Build history of the part. All positions in model axes, mm. A direction names the side the tool comes from. Give positions to 0.01 mm unless a question says otherwise; leave off trailing zeros. Order: outer loops, then holes, each group sorted by start corner. A loop starts at its lowest first (then second) coordinate and runs counter-clockwise, first axis right, second up. Notation, with made-up numbers: (49.5, 13) -> (68.5, 13) arc R11 cw to (68.5, 18) -> close; hole circle Ø11 at (-27, 19). An arc over 180 degrees is marked (long way). Write item = value, one per line. Start each with the question number.
from build123d import *

# Parameters (mm, degrees)
SKETCH013_R                          = 1.25
EXTRUDE009_DEPTH                     = 12
SKETCH012_R                          = 1.25
EXTRUDE008_DEPTH                     = 15
SKETCH011_W                          = 40
SKETCH011_H                          = 25
EXTRUDE007_DEPTH                     = 5
SKETCH010_W                          = 40
SKETCH010_H                          = 25
EXTRUDE006_DEPTH                     = 2
EXTRUDE004_DEPTH                     = 18
EXTRUDE004_ONTO_SKETCH007_ROLL_ANGLE = 90
SKETCH006_AS_DRAWN_R                 = 12.5
EXTRUDE003_DEPTH                     = 65
EXTRUDE003_ONTO_SKETCH006_ROLL_ANGLE = 90
EXTRUDE002_DEPTH                     = 60
EXTRUDE002_ONTO_SKETCH005_ROLL_ANGLE = 90
SKETCH004_R                          = 1.65
EXTRUDE_DEPTH                        = 40
SKETCH_AS_DRAWN_W                    = 30
SKETCH_AS_DRAWN_H                    = 70
EXTRUDE001_DEPTH                     = 60
EXTRUDE001_ONTO_SKETCH_ROLL_ANGLE    = 90


with BuildPart() as extrude009:
    # Sketch013 → Extrude009 (new body)
    with BuildSketch(Plane.XY.offset(15)):
        with Locations((11.5, 56.5)):
            Circle(SKETCH013_R)
        with Locations((-11.5, 56.5)):
            Circle(SKETCH013_R)
    extrude(amount=EXTRUDE009_DEPTH)


with BuildPart() as extrude008:
    # Sketch012 → Extrude008 (new body)
    with BuildSketch(Plane.XY.offset(70)):
        with Locations((0, 47)):
            Circle(SKETCH012_R)
        with Locations((11.5, 56.5)):
            Circle(SKETCH012_R)
        with Locations((-11.5, 56.5)):
            Circle(SKETCH012_R)
    extrude(amount=-EXTRUDE008_DEPTH)


with BuildPart() as extrude007:
    # Sketch011 → Extrude007 (new body)
    with BuildSketch(Plane(origin=(0, 35, 16), x_dir=(1, 0, 0), z_dir=(0, 0, 1))):
        with Locations((0, 20)):
            Rectangle(SKETCH011_W, SKETCH011_H)
    extrude(amount=-EXTRUDE007_DEPTH)


with BuildPart() as extrude006:
    # Sketch010 → Extrude006 (new body)
    with BuildSketch(Plane(origin=(0, 35, 70), x_dir=(1, 0, 0), z_dir=(0, 0, 1))):
        with Locations((0, 20)):
            Rectangle(SKETCH010_W, SKETCH010_H)
    extrude(amount=-EXTRUDE006_DEPTH)


with BuildPart() as extrude004:
    # Sketch007 as drawn → Extrude004 (new)
    with BuildSketch(Plane.XY):
        Polygon((17, 44), (7, 36), (7, 25), (17, 25), align=None)
        Polygon((-17, 44), (-7, 36), (-7, 25), (-17, 25), align=None)
    extrude(amount=-EXTRUDE004_DEPTH)


with BuildPart() as extrude004_1:
    # Extrude004 onto Sketch007 roll: moved
    add(extrude004.part.rotate(Axis((0, 0, 0), (1, 0, 0)), EXTRUDE004_ONTO_SKETCH007_ROLL_ANGLE))


with BuildPart() as extrude004_2:
    # Extrude004 onto Sketch007 placement: moved
    add(extrude004_1.part)


with BuildPart() as extrude003:
    # Sketch006 as drawn → Extrude003 (new)
    with BuildSketch(Plane.XY):
        with Locations((0, 50)):
            Circle(SKETCH006_AS_DRAWN_R)
    extrude(amount=-EXTRUDE003_DEPTH)


with BuildPart() as extrude003_1:
    # Extrude003 onto Sketch006 roll: moved
    add(extrude003.part.rotate(Axis((0, 0, 0), (1, 0, 0)), EXTRUDE003_ONTO_SKETCH006_ROLL_ANGLE))


with BuildPart() as extrude003_2:
    # Extrude003 onto Sketch006 placement: moved
    add(extrude003_1.part)


with BuildPart() as extrude002:
    # Sketch005 as drawn → Extrude002 (new)
    with BuildSketch(Plane.XY):
        with BuildLine():
            Line((2.5, 50), (2.5, 10))
            ThreePointArc((-2.5, 10), (0, 7.5), (2.5, 10))
            Line((-2.5, 10), (-2.5, 50))
            ThreePointArc((2.5, 50), (0, 52.5), (-2.5, 50))
        make_face()
    extrude(amount=-EXTRUDE002_DEPTH)


with BuildPart() as extrude002_1:
    # Extrude002 onto Sketch005 roll: moved
    add(extrude002.part.rotate(Axis((0, 0, 0), (1, 0, 0)), EXTRUDE002_ONTO_SKETCH005_ROLL_ANGLE))


with BuildPart() as extrude002_2:
    # Extrude002 onto Sketch005 placement: moved
    add(extrude002_1.part.moved(Location((0, -5, 0))))


with BuildPart() as extrude_cut_xy:
    # Sketch004 → Extrude (new body)
    with BuildSketch(Plane(origin=(0, 40, 0), x_dir=(0, 1, 0), z_dir=(1, 0, 0))):
        with Locations((-35.5, 32)):
            Circle(SKETCH004_R)
        with BuildLine():
            Line((7.5, 15), (30, 15))
            Line((30, 15), (30, 0))
            Line((30, 0), (0, 0))
            Line((0, 0), (0, 7.5))
            ThreePointArc((7.5, 15), (2.196699, 12.803301), (0, 7.5))
        make_face()
        with BuildLine():
            Line((7.5, 60), (30, 60))
            Line((30, 60), (30, 25))
            Line((30, 25), (7.5, 25))
            ThreePointArc((0, 32.5), (2.196699, 27.196699), (7.5, 25))
            Line((0, 32.5), (0, 52.5))
            ThreePointArc((7.5, 60), (2.196699, 57.803301), (0, 52.5))
        make_face()
        with BuildLine():
            Line((-10, 32), (-10, 0))
            Line((-10, 0), (-41, 0))
            Line((-41, 0), (-41, 28))
            Line((-41, 28), (-31, 28))
            Line((-31, 28), (-31, 32))
            ThreePointArc((-10, 32), (-20.5, 42.5), (-31, 32))
        make_face()
        with BuildLine():
            Line((-41, 80), (-5, 80))
            Line((-5, 80), (-5, 72.5))
            ThreePointArc((-12.5, 65), (-7.196699, 67.196699), (-5, 72.5))
            Line((-12.5, 65), (-41, 65))
            Line((-41, 65), (-41, 80))
        make_face()
    extrude(amount=EXTRUDE_DEPTH)


with BuildPart() as extrude_cut_xy_1:
    # Extrude placement: moved
    add(extrude_cut_xy.part.moved(Location((-20, 0, 0))))


with BuildPart() as cut007:
    # Sketch as drawn → Extrude001 (new)
    with BuildSketch(Plane.XY):
        with Locations((0, 35)):
            Rectangle(SKETCH_AS_DRAWN_W, SKETCH_AS_DRAWN_H)
    extrude(amount=-EXTRUDE001_DEPTH)


with BuildPart() as cut007_1:
    # Extrude001 onto Sketch roll: moved
    add(cut007.part.rotate(Axis((0, 0, 0), (1, 0, 0)), EXTRUDE001_ONTO_SKETCH_ROLL_ANGLE))


with BuildPart() as cut007_2:
    # Extrude001 onto Sketch placement: moved
    add(cut007_1.part)

    # Cut: cut extrude-cut-xy
    add(extrude_cut_xy_1.part, mode=Mode.SUBTRACT)

    # Cut001: cut Extrude002
    add(extrude002_2.part, mode=Mode.SUBTRACT)

    # Cut002: cut Extrude003
    add(extrude003_2.part, mode=Mode.SUBTRACT)

    # Cut003: cut Extrude004
    add(extrude004_2.part, mode=Mode.SUBTRACT)

    # Cut004: cut Extrude006
    add(extrude006.part, mode=Mode.SUBTRACT)

    # Cut005: cut Extrude007
    add(extrude007.part, mode=Mode.SUBTRACT)

    # Cut006: cut Extrude008
    add(extrude008.part, mode=Mode.SUBTRACT)

    # Cut007: cut Extrude009
    add(extrude009.part, mode=Mode.SUBTRACT)


solid = cut007_2.part
(1) Cut at D-D, the plane y = 4.5. Give the cut face in (x, z).
(2) Cut at C-C, the plane x = 4.5. Give the cut face in (y, z), plus the area to 3 significant figures.
(3) Flat gauge pins, fed straight in: P1, Ø3, axis at x = 5, z = 29.5, coming from the +Y side; P2, Ø6, axis at x = -0.5, y = 57, coming from the +Z side; P3, Ø8, axis at y = 8, z = 30.5, coming from the +X side. Where does each tip first touch, or does it go through?
(4) 3-axis set-ups, long thin cutter, end or side, ignore diameter. For faces 4 (the face through (0, 42.5, 69)), 5 (the face through (-9, 42.5, 15)), 6 (the face through (0, 14, 65)): which of +Z, -Z, +X, -X, +Y, -Y reach the whole face in a straight line?
(5) Wall check: line 1 (Y direction, x = 5, z = 32); line 2 (X direction, y = 39, z = 37); line 3 (Y direction, x = 11.5, z = 21.5). Give the ranges that are in metal, low to high. Write a range as [from, to].
(6) Cut at B-B, the plane z = 50. Give the cut face in (x, y).
(7) Cut at A-A, the plane y = 56.5. Give the cut face in (x, z), plus the area to 3 significant figures.
(8) Mould opens along Y. For faces 1 (the face through (-10.226, 23.307, 41.785)), 2 (the face through (-4, 51, 16)), 3 (the face through (-12.136, 43.266, 58.691)) say: released by +Y, released by -Y, zero draft, split by the parting line, or undercut.
Results:
q1.outline = (-15, 42.4) -> (-7, 36) -> (-7, 33.65) -> (-2.5, 33.65) -> (-2.5, 37.75) arc R12.5 cw (long way) to (2.5, 37.75) -> (2.5, 33.65) -> (7, 33.65) -> (7, 36) -> (15, 42.4) -> (15, 65) -> (-15, 65) -> close; (-7, 28) -> (-2.5, 28) -> (-2.5, 30.35) -> (-7, 30.35) -> close; (2.5, 28) -> (7, 28) -> (7, 30.35) -> (2.5, 30.35) -> close
q2.outline = (0, 28) -> (9, 28) -> (9, 32) arc R10.5 cw to (11.13, 38.34) -> (0, 38.34) -> close; (0, 61.66) -> (60, 61.66) -> (60, 68) -> (42.5, 68) -> (42.5, 70) -> (34.57, 70) arc R7.5 cw to (27.5, 65) -> (0, 65) -> close; (27.87, 38.34) arc R10.5 cw to (30, 32) -> (30, 0) -> (40, 0) -> (40, 7.5) arc R7.5 cw to (42.5, 13.09) -> (42.5, 16) -> (60, 16) -> (60, 25) -> (47.5, 25) arc R7.5 cw to (40, 32.5) -> (40, 38.34) -> close; hole circle Ø3.3 at (4.5, 32)
q2.area = 982 mm2
q3.P1 = 41.5
q3.P2 = 68
q3.P3 = 7
q4.face_4 = +Z, +X, -X, +Y
q4.face_5 = -Z, +X, -X, +Y
q4.face_6 = +Z, +X, -X, -Y
q5.line_1 = [0, 2.85], [6.15, 9], [30, 40.02]
q5.line_2 = [-15, -2.5], [2.5, 15]
q5.line_3 = [30, 55.25], [57.75, 60]
q6.outline = (-15, 0) -> (-12.5, 0) -> (-12.5, 40) -> (-15, 40) -> close; (12.5, 0) -> (15, 0) -> (15, 40) -> (12.5, 40) -> close
q7.outline = (-15, 16) -> (-12.75, 16) -> (-12.75, 25) -> (-15, 25) -> close; (-15, 60) -> (-12.75, 60) -> (-12.75, 68) -> (-15, 68) -> close; (-10.25, 16) -> (10.25, 16) -> (10.25, 25) -> (-10.25, 25) -> close; (-10.25, 60) -> (-7.5, 60) arc R12.5 cw to (7.5, 60) -> (10.25, 60) -> (10.25, 68) -> (-10.25, 68) -> close; (12.75, 16) -> (15, 16) -> (15, 25) -> (12.75, 25) -> close; (12.75, 60) -> (15, 60) -> (15, 68) -> (12.75, 68) -> close
q7.area = 399 mm2
q8.face_1 = undercut
q8.face_2 = zero draft
q8.face_3 = released by +Y
